Autodesk Inventor part; units mm, degrees
ref_plane "YZ Plane" through (0, 0, 0) normal (1, 0, 0) x (0, 1, 0)
ref_plane "XZ Plane" through (0, 0, 0) normal (0, 1, 0) x (-1, 0, 0)
ref_plane "XY Plane" through (0, 0, 0) normal (0, 0, 1) x (1, 0, 0)
sketch "Sketch1" plane through (0, 0, 0) normal (0, 1, 0) x (-1, 0, 0)
  circle A0 centre (0, 0) radius 58.5076
  circle A1 centre (0, 0) radius 64.8576
  dimension "d0" = 117.0153
  dimension "d1" = 129.7153
extrude "Extrusion1" add sketch "Sketch1" along normal blind 43.4975
sketch "Sketch2" plane through (0, 0, 0) normal (0, 1, 0) x (-1, 0, 0)
  circle A0 centre (0, 0) radius 51.562
  circle A1 centre (0, 0) radius 64.8576
  dimension "d4" = 103.124
  dimension "d5" = 129.7153
extrude "Extrusion2" add sketch "Sketch2" against normal blind 6.35
sketch "Sketch3" plane through (0, 0, 0) normal (0, 1, 0) x (-1, 0, 0)
  circle A0 centre (12.7, 12.7) radius 1.6256
  circle A1 centre (12.7, -12.7) radius 1.6256
  circle A2 centre (-12.7, 12.7) radius 1.6256
  circle A3 centre (-12.7, -12.7) radius 1.6256
  circle A4 centre (0, 0) radius 50.1447
  line L0 (53.4401, 17.2954) -> (47.8331, 15.0494)
  line L1 (0, 0) -> (53.4401, 17.2954)
  line L2 (43.7038, 24.586) -> (45.7401, 24.9855)
  line L3 (53.4401, 17.2954) -> (45.7401, 24.9855)
  line L4 (45.7401, 24.9855) -> (0, 0)
  dimension "d8" = 3.2512
  dimension "d9" = 3.2512
  dimension "d10" = 3.2512
  dimension "d11" = 3.2512
sketch "Sketch5" plane through (0, 0, 0) normal (0, 1, 0) x (-1, 0, 0)
  circle A0 centre (0, 0) radius 64.8576
  arc A1 (64.8576, 0) -> (44.4312, 47.2481) centre (0, 0) ccw
  arc A2 (50.9046, 0) -> (35.0064, 36.9572) centre (0, 0) ccw
  line L0 (35.0064, 36.9572) -> (44.4312, 47.2481)
  line L1 (50.9046, 0) -> (64.8576, 0)
  arc A3 (64.8576, 0) -> (44.4312, 47.2481) centre (0, 0) ccw
extrude "Extrusion3" cut sketch "Sketch5" against normal blind 7.62 contours L1 A2 L0 A0 picked at (59.6957, 6.2583)
sketch "Sketch10" plane through (0, 0, 0) normal (0, 0, 1) x (1, 0, 0)
  circle A0 centre (-15.0012, 25.7302) radius 3.2499
  point P0 (0, 0)
  dimension "d27" = 6.4999
extrude "Extrusion8" cut sketch "Sketch10" along normal mid plane 152.4
sketch "Sketch11" plane through (0, 0, 0) normal (0, 0, 1) x (1, 0, 0)
  circle A0 centre (15.0012, 25.7302) radius 3.2499
  point P0 (0, 0)
  dimension "d30" = 6.4999
extrude "Extrusion9" cut sketch "Sketch11" along normal mid plane 152.4
sketch "Sketch12" plane through (0, -6.35, 0) normal (0, -1, 0) x (1, 0, 0)
  line L0 (-58.5076, 0) -> (-64.8576, 0)
  line L1 (-64.8576, 0) -> (-49.4674, 0)
  line L2 (-49.4674, 0) -> (-49.4674, -12.7)
  line L3 (-49.4674, -12.7) -> (-64.8576, -12.7)
  line L4 (-64.8576, -12.7) -> (-64.8576, 0)
  point P0 (0, 0)
  dimension "d33" = 12.7
extrude "Extrusion10" cut sketch "Sketch12" against normal blind 6.35
sketch "Sketch13" plane through (0, -6.35, 0) normal (0, -1, 0) x (1, 0, 0)
  point P0 (0, 0)
sketch "Sketch14" plane through (0, -6.35, 0) normal (0, -1, 0) x (1, 0, 0)
  line L0 (-35.1204, 55.8851) -> (-25.6536, 41.7778)
  line L1 (-25.6536, 41.7778) -> (-33.019, 34.9455)
  line L2 (-44.4312, 47.2481) -> (-40.1421, 42.5648)
  line L3 (-44.4312, 47.2481) -> (-48.028, 43.8657)
  circle A0 centre (0, 0) radius 64.8576
  line L4 (-48.028, 43.8657) -> (-35.1204, 32.9693)
  line L5 (-35.1204, 32.9693) -> (-33.019, 34.9455)
  line L6 (-48.028, 43.8657) -> (-45.6028, 48.5109)
  line L7 (-45.6028, 48.5109) -> (-35.1204, 55.8851)
  dimension "d36" = 12.7
extrude "Extrusion11" cut sketch "Sketch14" against normal blind 6.35 contours L0 A0 L3 L6 L7 | L0 L1 L5 L4 A0 | A0 L4 L3 picked at (-33.3184, 42.2486)
properties part number "loader20190318_part2"
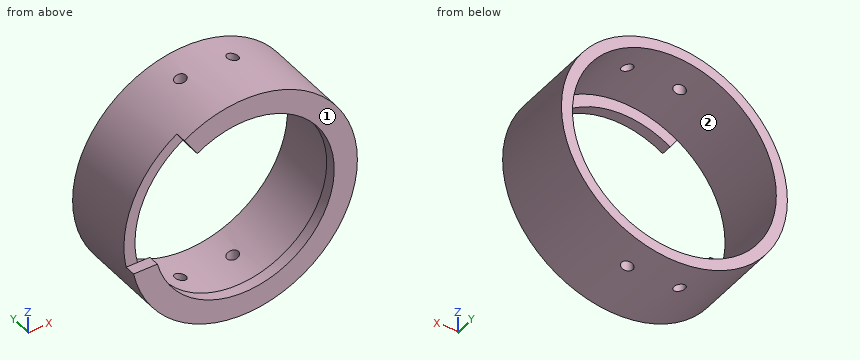
The listing builds one solid part. Answer for the finished solid, in the listing's coordinates (mm). Face numbers are marked on the shaded views. A direction names the side the tool comes from. Round coordinates to 2 decimals unless told otherwise and drop trailing zeros. Order: outer loops, then holes, each group sorted by start corner. A loop starts at its lowest first (then second) coordinate and runs counter-clockwise, first axis right, second up. Notation, with made-up numbers: (78, -13) - (134, -13) arc R9 ccw to (134, 3) - close; hole circle Ø1 at (21.5, -1.5). An arc over 180 degrees is marked (long way). Write item = value, one per line. Start each with the question number.
1) Given pin 1 (5 mm diameter, centred on x = 15, y = 25.73, fed in from +Z); pin 2 (7.5 mm diameter, centred on x = 15, y = 25.73, fed in from +Z); pin 3 (1 mm diameter, centred on y = 18, z = -32, fed in from -X); pin 4 (5 mm diameter, centred on y = 5.5, z = -32, fed in from -X), each flat-ended and moving along its own axis, determine where each tip first touches the part or whether it passes through.
2) For the marked faces 1 and 2, determine the directions among +Z, -Z, +X, -X, +Y, -Y from which every point of the face is accessible in a straight line to the end or side of a thin tool.
3) Section B-B, the plane z = 0 is taken. Write down the section's boundary in (x, y), plus the area to 3 significant figures.
4) Section D-D, the plane z = -19 is taken. Write down the section's boundary in (x, y), plus the area to 3 significant figures.
5) Section C-C, the plane y = 4 is taken. Write down the section's boundary in (x, z).
6) Straight lines are drawn through the part: L1, parallel to Z at x = 0, y = -2; L2, parallel to X at y = 32.5, z = -1.5; L3, parallel to Z at x = 0.5, y = 21. For each, find the intervals that lie inside material, in ascending order.
7) Section A-A, the plane x = 0 is taken. Write down the section's boundary in (y, z), plus the area to 3 significant figures.
Results list:
q1.pin_1 = through
q1.pin_2 = 63.87
q1.pin_3 = -56.69
q1.pin_4 = -57.76
q2.face_1 = +Z, -Z, +X, -X, -Y
q2.face_2 = +Y
q3.outline = (-64.86, 0) - (-58.51, 0) - (-58.51, 43.5) - (-64.86, 43.5) - close; (51.56, -6.35) - (64.86, -6.35) - (64.86, 43.5) - (58.51, 43.5) - (58.51, 0) - (51.56, 0) - close
q3.area = 637 mm^2
q4.outline = (-62.01, -6.35) - (-47.93, -6.35) - (-47.93, 0) - (-55.34, 0) - (-55.34, 43.5) - (-62.01, 43.5) - close; (47.93, -6.35) - (62.01, -6.35) - (62.01, 43.5) - (55.34, 43.5) - (55.34, 0) - (47.93, 0) - close
q4.area = 760 mm^2
q5.outline = circle Ø129.72 at (0, 0); hole circle Ø117.02 at (0, 0)
q6.L1 = -64.86 to -51.56, 51.56 to 64.86
q6.L2 = -64.84 to -58.49, 58.49 to 64.84
q6.L3 = -64.86 to -58.51, 58.51 to 64.86
q7.outline = (-6.35, -64.86) - (43.5, -64.86) - (43.5, -58.51) - (0, -58.51) - (0, -51.56) - (-6.35, -51.56) - close; (-6.35, 51.56) - (0, 51.56) - (0, 58.51) - (43.5, 58.51) - (43.5, 64.86) - (-6.35, 64.86) - close
q7.area = 721 mm^2
